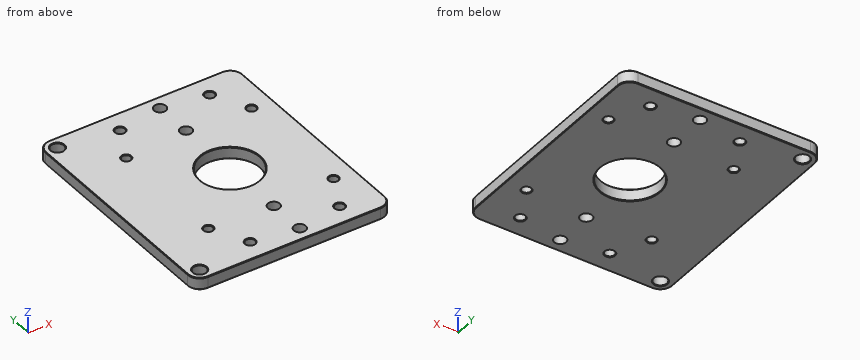
```python
from build123d import *

# Parameters (mm, degrees)
SKETCH_2_W                  = 38
SKETCH_2_H                  = 39
EXTRUDE_1_DEPTH             = 2
CHAMFER_3_SIZE              = 1
SKETCH_7_R                  = 5
CUT_EXTRUDE_3_DEPTH         = 10
SKETCH_8_W                  = 2
SKETCH_8_H                  = 39
CUT_EXTRUDE_4_DEPTH         = 10
FILLET_3_R                  = 2
SKETCH_9_R                  = 2
EXTRUDE_1_2_DEPTH           = 23
SKETCH_10_W                 = 3
SKETCH_10_H                 = 39
CUT_EXTRUDE_1_DEPTH         = 10
FILLET_5_R                  = 2
CHAMFER_5_SIZE              = 0.5
HOLE_WIZARD_M2_1_D          = 1.6
HOLE_WIZARD_2_2_2_2_1_D     = 2.2
HOLE_WIZARD_2_2_2_2_1_DEPTH = 114
HOLE_WIZARD_2_2_2_2_1_TIP   = 0.660946681
SKETCH_24_W                 = 68.041100534
SKETCH_24_H                 = 56.84151123
CUT_EXTRUDE_3_2_DEPTH       = 95
HOLE_WIZARD_1_5_1_5_1_D     = 1.5
HOLE_WIZARD_1_5_1_5_1_DEPTH = 43
HOLE_WIZARD_1_5_1_5_1_TIP   = 0.450645464
CHAMFER_6_SIZE              = 0.1
CHAMFER_7_SIZE              = 0.1
HOLE_WIZARD_2_0_2_1_D       = 2


with BuildPart() as part:
    # 草图2 → Extrude 1 (new body)
    with BuildSketch(Plane.XY):
        Rectangle(SKETCH_2_W, SKETCH_2_H)
    extrude(amount=EXTRUDE_1_DEPTH)

    # 倒角3
    chamfer_3_edges = [part.edges().sort_by_distance(p)[0] for p in [
        (-19, 19.5, 1),
        (-19, -19.5, 1),
    ]]
    chamfer(chamfer_3_edges, length=CHAMFER_3_SIZE)

    # 草图7 → Cut-Extrude 3 (cut)
    with BuildSketch(Plane.XY.offset(2)):
        with Locations((2, 0)):
            Circle(SKETCH_7_R)
    extrude(amount=-CUT_EXTRUDE_3_DEPTH, mode=Mode.SUBTRACT)

    # 草图8 → 拉伸4 (cut)
    with BuildSketch(Plane.XY.offset(2)):
        with Locations((-18, 0)):
            Rectangle(SKETCH_8_W, SKETCH_8_H)
    extrude(amount=-CUT_EXTRUDE_4_DEPTH, mode=Mode.SUBTRACT)

    # 圆角3
    fillet_3_edges = [part.edges().sort_by_distance(p)[0] for p in [
        (-17, 19.5, 1),
        (-17, -19.5, 1),
    ]]
    fillet(fillet_3_edges, radius=FILLET_3_R)

    # 草图9 → Extrude 1 2 (add)
    with BuildSketch(Plane.XY.offset(2)):
        with Locations((-15, 17.5)):
            Circle(SKETCH_9_R)
        with Locations((-15, -17.5)):
            Circle(SKETCH_9_R)
    extrude_1_2 = extrude(amount=EXTRUDE_1_2_DEPTH)

    # 镜向1: Extrude 1 2 across plane
    add(extrude_1_2.mirror(Plane.ZX))

    # 草图10 → 切除-拉伸1 (cut)
    with BuildSketch(Plane(origin=(0, 0, 0), x_dir=(-1, 0, 0), z_dir=(0, 0, -1))):
        with Locations((-17.5, 0)):
            Rectangle(SKETCH_10_W, SKETCH_10_H)
    extrude(amount=-CUT_EXTRUDE_1_DEPTH, mode=Mode.SUBTRACT)

    # 圆角5
    fillet_5_edges = [part.edges().sort_by_distance(p)[0] for p in [
        (16, -19.5, 1),
        (16, 19.5, 1),
    ]]
    fillet(fillet_5_edges, radius=FILLET_5_R)

    # 倒角5
    chamfer_5_edges = [part.edges().sort_by_distance(p)[0] for p in [
        (-17, 17.5, 25),
        (-17, -17.5, 25),
    ]]
    chamfer(chamfer_5_edges, length=CHAMFER_5_SIZE)

    # M2 螺纹孔1 (through all)
    with Locations(Plane(origin=(9.5, 16, 0), x_dir=(-1, 0, 0), z_dir=(0, 0, -1))):
        with Locations((0, 0), (15, 0), (0, -32), (15, -32)):
            Hole(HOLE_WIZARD_M2_1_D / 2)

    # Ø2.2 (2.2) 直径孔1
    with Locations(Plane(origin=(-15, 17.5, 25), x_dir=(1, 0, 0), z_dir=(0, 0, 1))):
        with Locations((0, 0), (0, -35)):
            Hole(HOLE_WIZARD_2_2_2_2_1_D / 2, depth=HOLE_WIZARD_2_2_2_2_1_DEPTH)
            with Locations((0, 0, -(HOLE_WIZARD_2_2_2_2_1_DEPTH + HOLE_WIZARD_2_2_2_2_1_TIP / 2))):  # 118° drill point
                Cone(0, HOLE_WIZARD_2_2_2_2_1_D / 2, HOLE_WIZARD_2_2_2_2_1_TIP, mode=Mode.SUBTRACT)

    # 草图24 → Cut-Extrude 3 2 (cut)
    with BuildSketch(Plane.XY.offset(2)):
        Rectangle(SKETCH_24_W, SKETCH_24_H)
    extrude(amount=CUT_EXTRUDE_3_2_DEPTH, mode=Mode.SUBTRACT)

    # Ø1.5 (1.5) 直径孔1
    with Locations(Plane(origin=(12.5, 10.1, 0), x_dir=(-1, 0, 0), z_dir=(0, 0, -1))):
        with Locations((0, 0), (21, 0), (21, -20.2), (0, -20.2)):
            Hole(HOLE_WIZARD_1_5_1_5_1_D / 2, depth=HOLE_WIZARD_1_5_1_5_1_DEPTH)
            with Locations((0, 0, -(HOLE_WIZARD_1_5_1_5_1_DEPTH + HOLE_WIZARD_1_5_1_5_1_TIP / 2))):  # 118° drill point
                Cone(0, HOLE_WIZARD_1_5_1_5_1_D / 2, HOLE_WIZARD_1_5_1_5_1_TIP, mode=Mode.SUBTRACT)

    # 倒角6
    chamfer_6_edges = [part.edges().sort_by_distance(p)[0] for p in [
        (-13.9, 17.5, 0),
        (-13.9, -17.5, 0),
        (8.7, 16, 0),
        (-6.3, 16, 0),
        (8.7, -16, 0),
        (15.414213562, 18.914213562, 0),
        (-0.5, 19.5, 0),
        (-16.414213562, 18.914213562, 0),
        (-17, 0, 0),
        (-16.414213562, -18.914213562, 0),
        (-0.5, -19.5, 0),
        (15.414213562, -18.914213562, 0),
        (16, 0, 0),
        (-3, 0, 0),
        (-6.3, -16, 0),
        (11.75, -10.1, 0),
        (-9.25, -10.1, 0),
        (-9.25, 10.1, 0),
        (11.75, 10.1, 0),
    ]]
    chamfer(chamfer_6_edges, length=CHAMFER_6_SIZE)

    # 倒角7
    chamfer_7_edges = [part.edges().sort_by_distance(p)[0] for p in [
        (-13.9, -17.5, 2),
        (-13.9, 17.5, 2),
        (8.7, 16, 2),
        (-6.3, 16, 2),
        (8.7, -16, 2),
        (-6.3, -16, 2),
        (-16.414213562, -18.914213562, 2),
        (-17, 0, 2),
        (-13.9, 17.5, 2),
        (-0.5, 19.5, 2),
        (15.414213562, 18.914213562, 2),
        (16, 0, 2),
        (15.414213562, -18.914213562, 2),
        (-0.5, -19.5, 2),
        (-3, 0, 2),
        (11.75, -10.1, 2),
        (-9.25, -10.1, 2),
        (-9.25, 10.1, 2),
        (11.75, 10.1, 2),
    ]]
    chamfer(chamfer_7_edges, length=CHAMFER_7_SIZE)

    # Ø2.0 (2) 直径孔1 (through all)
    with Locations(Plane(origin=(2, 10.8, 0), x_dir=(-1, 0, 0), z_dir=(0, 0, -1))):
        with Locations((0, 0), (0, 6.4)):
            hole_wizard_2_0_2_1 = Hole(HOLE_WIZARD_2_0_2_1_D / 2)

    # 镜向3: Ø2.0 (2) 直径孔1 across plane
    add(hole_wizard_2_0_2_1.mirror(Plane.ZX), mode=Mode.SUBTRACT)


solid = part.part
```
Design review of the part built by this model. Coordinates are the model's own, in mm. Coordinates: 2 decimals unless noted, no trailing zeros. Order: outer loops, then holes, each group sorted by start corner. A loop starts at its lowest first (then second) coordinate and runs counter-clockwise, first axis right, second up. Notation, with made-up numbers: (82, 7) - (141, 7) arc R27 cw to (141, 27) - close; hole circle Ø5 at (87, -18). An arc over 180 degrees is marked (long way). Answer in a Markdown table with one row per item.
(1) Consider section A-A on y = 0. State the section outline as (x, z) points.
Checked values:
| item | result |
|---|---|
| outline | (-17, 0.1) - (-16.9, 0) - (-3.1, 0) - (-3, 0.1) - (-3, 1.9) - (-3.1, 2) - (-16.9, 2) - (-17, 1.9) - close; (7, 0.1) - (7.1, 0) - (15.9, 0) - (16, 0.1) - (16, 1.9) - (15.9, 2) - (7.1, 2) - (7, 1.9) - close |
(2) Consider section B-B on x = 9.5. State the section outline as (y, z) points.
Checked values:
| item | result |
|---|---|
| outline | (-19.5, 0.1) - (-19.4, 0) - (-16.9, 0) - (-16.8, 0.1) - (-16.8, 1.9) - (-16.9, 2) - (-19.4, 2) - (-19.5, 1.9) - close; (-15.2, 0.1) - (-15.1, 0) - (15.1, 0) - (15.2, 0.1) - (15.2, 1.9) - (15.1, 2) - (-15.1, 2) - (-15.2, 1.9) - close; (16.8, 0.1) - (16.9, 0) - (19.4, 0) - (19.5, 0.1) - (19.5, 1.9) - (19.4, 2) - (16.9, 2) - (16.8, 1.9) - close |
(3) Wall thickness on line 1 along Y through (x, z) = (9.5, 0.95); line 2 along Y through (x, z) = (12.5, 1.45); line 3 along Y through (x, z) = (2, 0.65): over which ranges is each line inside the solid? List them lowest first. Write a range as from..to.
Checked values:
| item | result |
|---|---|
| line 1 | -19.5..-16.8, -15.2..15.2, 16.8..19.5 |
| line 2 | -19.5..-10.85, -9.35..9.35, 10.85..19.5 |
| line 3 | -19.5..-18.2, -16.2..-11.8, -9.8..-5, 5..9.8, 11.8..16.2, 18.2..19.5 |
(4) Consider section C-C on z = 0.6. Give the number of separate pieces and of enclosed holes in the cut face, plus the area to 3 significant figures.
Checked values:
| item | result |
|---|---|
| separate pieces | 1 |
| enclosed holes | 15 |
| area | 1,170 mm^2 |
(5) Clearance check with a flat-ended pin moving along its axis: pin 1 (0.9 mm diameter, centred on x = -8.5, y = 10.1, fed in from -Z). State where the tip first meets the part, or that it passes through.
Checked values:
| item | result |
|---|---|
| pin 1 | through |
